from build123d import *

# Parameters (mm, degrees)
BOSS_EXTRUDE1_DEPTH           = 28
SHELL2_T                      = -1
BOSS_EXTRUDE2_DEPTH           = 4.5
CUT_EXTRUDE1_DEPTH            = 4.5
SKETCH8_R                     = 1.2
CUT_EXTRUDE2_DEPTH            = 24.5
SKETCH9_R                     = 1.2
CUT_EXTRUDE3_DEPTH            = 24.5
SKETCH10_R                    = 1.2
CUT_EXTRUDE4_DEPTH            = 24.5
BOSS_EXTRUDE3_DEPTH           = 10
BOSS_EXTRUDE4_DEPTH           = 19.253744603
CUT_EXTRUDE5_DEPTH            = 10
CUT_EXTRUDE6_DEPTH            = 10
CUT_EXTRUDE7_DEPTH            = 10
BOSS_EXTRUDE5_DEPTH           = 19.253744603
CUT_EXTRUDE8_DEPTH            = 10
BOSS_EXTRUDE6_DEPTH           = 1
SKETCH23_R                    = 4.75
CUT_EXTRUDE9_DEPTH            = 1
SKETCH24_R                    = 4.755
BOSS_EXTRUDE7_DEPTH           = 6.2
BOSS_EXTRUDE7_TAPER           = -2
BOSS_EXTRUDE7_OTHER_WAY_DEPTH = 0.674501
SKETCH28_R                    = 4.245
CUT_EXTRUDE10_DEPTH           = 76
CUT_EXTRUDE10_DRAFT           = 2


with BuildPart() as part:
    # Sketch3 → Boss-Extrude1 (new body)
    with BuildSketch(Plane(origin=(0, 0, 0), x_dir=(1, 0, 0), z_dir=(0, 0.6691306063588569, 0.7431448254773955))):
        Polygon((-9, 0), (9, 0), (26.698804633, 8.185494155), (29.511256471, 2.104366409), (11.812451838, -6.081127746), (-11.812451838, -6.081127746), (-29.511256471, 2.104366409), (-26.698804633, 8.185494155), align=None)
    extrude(amount=BOSS_EXTRUDE1_DEPTH)

    # Shell2
    shell2_openings = [part.faces().sort_by_distance(p)[0] for p in [
        (20.661854154, 7.890173684, 11.734513919),
        (0, 4.848669872, 14.473096253),
        (-20.661854154, 7.890173684, 11.734513919),
    ]]
    offset(amount=SHELL2_T, openings=shell2_openings, kind=Kind.INTERSECTION)

    # Sketch5 → Boss-Extrude2 (add)
    with BuildSketch(Plane(origin=(0, 0.6691306063588575, 0.7431448254773962), x_dir=(1, 0, 0), z_dir=(0, 0.669130606358857, 0.7431448254773954))):
        Polygon((-28.603625464, 1.684597478), (-28.183856533, 2.592228485), (-11.392682907, -5.173496739), (11.392682907, -5.173496739), (28.183856533, 2.592228485), (28.603625464, 1.684597478), (11.812451838, -6.081127746), (-11.812451838, -6.081127746), align=None)
    extrude(amount=BOSS_EXTRUDE2_DEPTH)

    # Sketch6 → Cut-Extrude1 (cut)
    with BuildSketch(Plane(origin=(0, 0.6691306063588575, 0.7431448254773962), x_dir=(1, 0, 0), z_dir=(0, 0.669130606358857, 0.7431448254773954))):
        Polygon((9.220047236, -1), (26.210942557, 6.858094217), (28.183856533, 2.592228485), (11.392682907, -5.173496739), (-11.392682907, -5.173496739), (-28.183856533, 2.592228485), (-26.210942557, 6.858094217), (-9.220047236, -1), align=None)
    extrude(amount=-CUT_EXTRUDE1_DEPTH, mode=Mode.SUBTRACT)

    # Sketch8 → Cut-Extrude2 (cut)
    with BuildSketch(Plane(origin=(0, 0, 0), x_dir=(1, 0, 0), z_dir=(0, 0.7431448254773954, -0.669130606358857))):
        with Locations(Location((5.93, -3.91, 0), (0, 0, 270))):
            Circle(SKETCH8_R)
        with Locations(Location((-5.93, -3.91, 0), (0, 0, 270))):
            Circle(SKETCH8_R)
        with Locations(Location((5.93, -23.63, 0), (0, 0, 270))):
            Circle(SKETCH8_R)
        with Locations(Location((-5.93, -23.63, 0), (0, 0, 270))):
            Circle(SKETCH8_R)
    extrude(amount=-CUT_EXTRUDE2_DEPTH, mode=Mode.SUBTRACT)

    # Sketch9 → Cut-Extrude3 (cut)
    with BuildSketch(Plane(origin=(1.585853599, -2.548212155, 2.29442053), x_dir=(0.907631006833055, 0.3119491089708923, -0.2808802393324979), z_dir=(-0.4197689310027779, 0.6745012861708234, -0.6073236859523018))):
        with Locations(Location((23.758679061, -3.91, 0), (0, 0, 270))):
            Circle(SKETCH9_R)
        with Locations(Location((11.738679061, -3.91, 0), (0, 0, 270))):
            Circle(SKETCH9_R)
        with Locations(Location((23.758679061, -23.97, 0), (0, 0, 270))):
            Circle(SKETCH9_R)
        with Locations(Location((11.738679061, -23.97, 0), (0, 0, 270))):
            Circle(SKETCH9_R)
    extrude(amount=-CUT_EXTRUDE3_DEPTH, mode=Mode.SUBTRACT)

    # Sketch10 → Cut-Extrude4 (cut)
    with BuildSketch(Plane(origin=(-1.585853599, -2.548212155, 2.29442053), x_dir=(0.907631006833055, -0.3119491089708923, 0.2808802393324979), z_dir=(0.4197689310027779, 0.6745012861708234, -0.6073236859523018))):
        with Locations(Location((-11.738679061, -3.91, 0), (0, 0, 270))):
            Circle(SKETCH10_R)
        with Locations(Location((-23.758679061, -3.91, 0), (0, 0, 270))):
            Circle(SKETCH10_R)
        with Locations(Location((-11.738679061, -23.93, 0), (0, 0, 270))):
            Circle(SKETCH10_R)
        with Locations(Location((-23.758679061, -23.93, 0), (0, 0, 270))):
            Circle(SKETCH10_R)
    extrude(amount=-CUT_EXTRUDE4_DEPTH, mode=Mode.SUBTRACT)

    # Sketch11 → Boss-Extrude3 (add, along a direction that is not the sketch's normal)
    with BuildSketch(Plane(origin=(0, 0, 0), x_dir=(-1, 0, 0), z_dir=(0, -0.669130606358857, -0.7431448254773954))):
        Polygon((-11.812451838, -6.081127746), (-11.392682907, -5.173496739), (11.392682907, -5.173496739), (11.812451838, -6.081127746), align=None)
        Polygon((-9.220047236, -1), (-9, 0), (9, 0), (9.220047236, -1), align=None)
    extrude(amount=BOSS_EXTRUDE3_DEPTH, dir=(0, 0, -1))

    # Sketch12 → Boss-Extrude4 (add, along a direction that is not the sketch's normal)
    with BuildSketch(Plane(origin=(0, 0, 0), x_dir=(-1, 0, 0), z_dir=(0, -0.669130606358857, -0.7431448254773954))):
        Polygon((-11.812451838, -6.081127746), (-11.392682907, -5.173496739), (-28.183856533, 2.592228485), (-26.210942557, 6.858094217), (-9.220047236, -1), (-9, 0), (-26.698804633, 8.185494155), (-29.511256471, 2.104366409), align=None)
    extrude(amount=BOSS_EXTRUDE4_DEPTH, dir=(-0.9192395760563791, -0.3159389272983625, -0.2349067815735609))

    # Sketch14 → Cut-Extrude5 (cut, along a direction that is not the sketch's normal)
    with BuildSketch(Plane(origin=(0, -4.972609477, -5.522642316), x_dir=(-1, 0, 0), z_dir=(0, -0.6691306063588573, -0.743144825477395))):
        Polygon((4.148710376, 0.610178318), (1.766447359, 0.610178318), (8.478757397, -2.494188091), (8.698804633, -1.494188091), align=None)
    extrude(amount=-CUT_EXTRUDE5_DEPTH, dir=(0, 0, -1), mode=Mode.SUBTRACT)

    # Sketch15 → Cut-Extrude6 (cut, along a direction that is not the sketch's normal)
    with BuildSketch(Plane(origin=(0, -4.972609477, -5.522642316), x_dir=(-1, 0, 0), z_dir=(0, -0.6691306063588573, -0.743144825477395))):
        Polygon((-11.812451838, 0.610178318), (-9.430188821, 0.610178318), (6.306121727, -6.66768483), (5.886352796, -7.575315837), align=None)
    extrude(amount=-CUT_EXTRUDE6_DEPTH, dir=(0, 0, -1), mode=Mode.SUBTRACT)

    # Sketch16 → Cut-Extrude7 (cut, along a direction that is not the sketch's normal)
    with BuildSketch(Plane(origin=(0, -4.972609477, -5.522642316), x_dir=(-1, 0, 0), z_dir=(0, -0.6691306063588573, -0.743144825477395))):
        Polygon((-0.196046727, 1.517809325), (2.18621629, 1.517809325), (-6.837784219, 5.691306064), (-8.512137924, 5.363906126), align=None)
    extrude(amount=-CUT_EXTRUDE7_DEPTH, dir=(0, 0, -1), mode=Mode.SUBTRACT)

    # Sketch18 → Boss-Extrude5 (add, along a direction that is not the sketch's normal)
    with BuildSketch(Plane(origin=(0, 0, 0), x_dir=(-1, 0, 0), z_dir=(0, -0.669130606358857, -0.7431448254773954))):
        Polygon((9, 0), (9.220047236, -1), (26.210942557, 6.858094217), (28.183856533, 2.592228485), (11.392682907, -5.173496739), (11.812451838, -6.081127746), (29.511256471, 2.104366409), (26.698804633, 8.185494155), align=None)
    extrude(amount=BOSS_EXTRUDE5_DEPTH, dir=(0.9192395760563791, -0.3159389272983624, -0.2349067815735607))

    # Sketch19 → Cut-Extrude8 (cut, along a direction that is not the sketch's normal)
    with BuildSketch(Plane(origin=(0, -4.972609477, -5.522642316), x_dir=(-1, 0, 0), z_dir=(0, -0.6691306063588573, -0.743144825477395))):
        Polygon((6.837784219, 5.691306064), (8.512137924, 5.363906126), (0.196046727, 1.517809325), (-2.18621629, 1.517809325), align=None)
        Polygon((-4.148710376, 0.610178318), (-1.766447359, 0.610178318), (-8.478757397, -2.494188091), (-8.698804633, -1.494188091), align=None)
        Polygon((9.430188821, 0.610178318), (11.812451838, 0.610178318), (-5.886352796, -7.575315837), (-6.306121727, -6.66768483), align=None)
    extrude(amount=-CUT_EXTRUDE8_DEPTH, dir=(0, 0, -1), mode=Mode.SUBTRACT)

    # Sketch20 → Boss-Extrude6 (add)
    with BuildSketch(Plane(origin=(0, -4.972609477, -5.522642316), x_dir=(-1, 0, 0), z_dir=(0, -0.6691306063588573, -0.743144825477395))):
        Polygon((-11.812451838, 0.610178318), (-9, 6.691306064), (9, 6.691306064), (11.812451838, 0.610178318), align=None)
    extrude(amount=-BOSS_EXTRUDE6_DEPTH)

    # Sketch23 → Cut-Extrude9 (cut)
    with BuildSketch(Plane.XZ.offset(4.519158617)):
        with Locations((0.002451838, -0.930931304)):
            Circle(SKETCH23_R)
    extrude(amount=-CUT_EXTRUDE9_DEPTH, mode=Mode.SUBTRACT)

    # Sketch24 → Boss-Extrude7 (add)
    with BuildSketch(Plane.XZ.offset(4.519158617)):
        with Locations((0.002451838, -0.930931304)):
            Circle(SKETCH24_R)
    extrude(amount=BOSS_EXTRUDE7_DEPTH, taper=BOSS_EXTRUDE7_TAPER)

    # Sketch24 → Boss-Extrude7 other way (add)
    with BuildSketch(Plane.XZ.offset(4.519158617)):
        with Locations((0.002451838, -0.930931304)):
            Circle(SKETCH24_R)
    extrude(amount=-BOSS_EXTRUDE7_OTHER_WAY_DEPTH)


with BuildPart() as cut_extrude10_tool:
    # Sketch28 → Cut-Extrude10 (with draft: the straight prism first)
    with BuildSketch(Plane(origin=(0, -3.844657331, 0), x_dir=(1, 0, 0), z_dir=(0, 1, 0))):
        with Locations((0.002451838, 0.930931304)):
            Circle(SKETCH28_R)
    extrude(amount=-CUT_EXTRUDE10_DEPTH)
    # Cut-Extrude10: the draft: its side faces are tilted about the plane it starts from
    cut_extrude10_sides = [cut_extrude10_tool.faces().sort_by_distance(p)[0] for p in [
        (-4.242548162, -41.844657331, -0.930931304),
    ]]
    draft(cut_extrude10_sides, Plane(origin=(0, -3.844657331, 0), x_dir=(1, 0, 0), z_dir=(0, 1, 0)), CUT_EXTRUDE10_DRAFT)


with BuildPart() as part_1:
    add(part.part)

    # Cut-Extrude10: cut by cut_extrude10_tool
    add(cut_extrude10_tool.part, mode=Mode.SUBTRACT)


solid = part_1.part
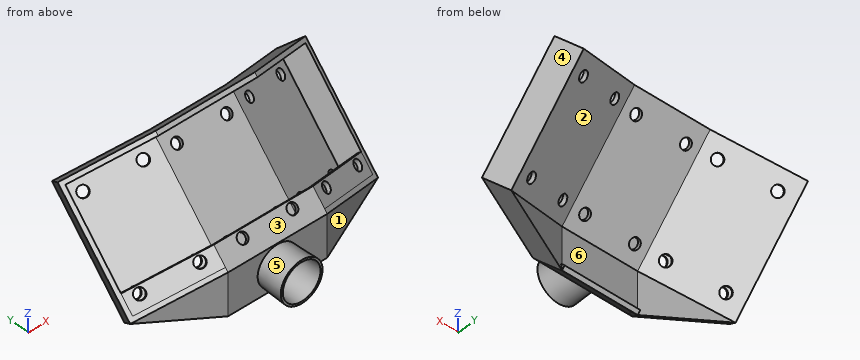
Can you work these out from the model? Positions are in its coordinate system, mm. Face numbers are marked on the shaded views. A direction names the side the tool comes from. Give positions to 0.01 mm unless a question says otherwise; leave off trailing zeros. Loops run counter-clockwise (first coordinate to the right, second up) from the corner with the lowest first, then second, coordinate; pieces in that order, holes last. Notation, with made-up numbers: (19, 52) -> (74, 52) arc R12 ccw to (74, 67) -> close; hole circle Ø7 at (21.5, 30). An arc over 180 degrees is marked (long way). Return JSON: item names as keys, results as strings.
Q1. For pin 1 Ø9.5 at (x, z) = (4.5, -2.5) entering from +Y; pin 2 Ø1 at (x, z) = (15, -5.5) entering from -Y; pin 3 Ø4.5 at (x, z) = (-0.5, -2) entering from -Y, each with a flat end and sliding along its axis, tell me the tip position at first contact or that it passes through.
Checks:
{"pin 1": "stops at y = 2.03", "pin 2": "stops at y = -3.57", "pin 3": "stops at y = -0.74"}
Q2. I want a section at B-B, the plane z = 11.5. List the corners of the cut face in (x, y) for me.
Checks:
{"outline": "(-29.51, 13.19) -> (-28.6, 12.62) -> (-26.21, 19.58) -> (-9.22, 9.01) -> (9.22, 9.01) -> (26.21, 19.58) -> (28.6, 12.62) -> (29.51, 13.19) -> (26.7, 21.37) -> (9, 10.35) -> (-9, 10.35) -> (-26.7, 21.37) -> close"}
Q3. We'd pull the mould along X, two halves only. Please class the marked faces 1, 2 and 3: released by +X, released by -X, zero draft, split by the parting line, or undercut.
Checks:
{"face 1": "released by +X", "face 2": "undercut", "face 3": "zero draft"}
Q4. I want a section at C-C, the plane x = 20. List the corners of the cut face in (y, z) for me, then the cut area to 3 significant figures.
Checks:
{"outline": "(-1.71, -3.84) -> (3.78, -7.19) -> (3.78, -3.4) -> (22.52, 17.4) -> (17.03, 22.34) -> (16.36, 21.6) -> (21.03, 17.4) -> (2.96, -2.67) -> (2.96, -6.18) -> (-0.89, -3.83) -> (-0.89, 0.8) -> (2.79, 4.89) -> (1.98, 5.62) -> (-1.71, 1.54) -> close", "area": "52.7 mm2"}
Q5. I want a section at A-A, the plane y = 22.5. List the corners of the cut face in (x, z) for me, then the cut area to 3 significant figures.
Checks:
{"outline": "(-28.14, 17.42) -> (-26.7, 12.76) -> (-19.95, 17.42) -> close; (19.95, 17.42) -> (26.7, 12.76) -> (28.14, 17.42) -> close; hole (-26.62, 16.07) -> (-26.21, 14.74) -> (-24.28, 16.07) -> close; hole (24.28, 16.07) -> (26.21, 14.74) -> (26.62, 16.07) -> close", "area": "35.1 mm2"}
Q6. I want a section at D-D, the plane y = -8. List the corners of the cut face in (x, z) for me.
Checks:
{"outline": "circle Ø9.75 at (0, -0.93); hole circle Ø8.78 at (0, -0.93)"}
Q7. I need wall thicknesses on probe 1 along X at (y, z) = (6, 6.5); probe 2 along X at (y, z) = (23.5, 16); probe 3 along Z at (x, y) = (-25.5, 4.5). Which ranges of each line are inside material? Lowest first, please.
Checks:
{"probe 1": "x = -11.62 to -9.24, 9.24 to 11.62", "probe 2": "x = -27.36 to -23.61, 23.61 to 27.36", "probe 3": "z = -5.07 to -4.56, 2.98 to 3.35"}
Q8. On a 3-axis mill with a long thin cutter (end or side, diameter ignored), from which of +Z, -Z, +X, -X, +Y, -Y can I reach the whole of each face in a straight line? I mean the marked faces 4, 5 and 6. Say none if no direction works.
Checks:
{"face 4": "-Z, +X, +Y", "face 5": "none", "face 6": "+Y"}
